Build history of the part. All positions in model axes, mm. Face numbers are marked on the shaded views. Coordinates: 2 decimals unless noted, no trailing zeros.
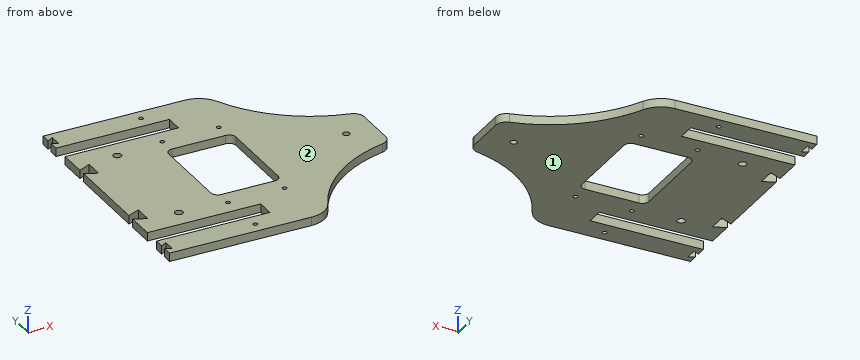
Autodesk Inventor part; units mm, degrees
ref_plane "YZ Plane" through (0, 0, 0) normal (1, 0, 0) x (0, 1, 0)
ref_plane "XZ Plane" through (0, 0, 0) normal (0, 1, 0) x (-1, 0, 0)
ref_plane "XY Plane" through (0, 0, 0) normal (0, 0, 1) x (1, 0, 0)
sketch "Boceto1" plane through (0, 0, 0) normal (0, 0, 1) x (1, 0, 0)
  line L0 (0.0213, 161.5) -> (84.4213, 161.5)
  line L1 (0.0213, 180) -> (0.0213, 172.7)
  line L2 (0.0213, 161.5) -> (0.0213, 168.8)
  line L3 (4.5413, 170.75) -> (4.5413, 175.3)
  line L4 (4.5413, 175.3) -> (0.0213, 172.7)
  line L5 (4.5413, 170.75) -> (4.5413, 166.2)
  line L6 (4.5413, 166.2) -> (0.0213, 168.8)
  line L7 (0.0213, 161.5) -> (84.4213, 161.5)
  line L8 (84.4213, 161.5) -> (84.4213, 148.5)
  line L9 (84.4213, 148.5) -> (0.0213, 148.5)
  line L10 (0.0213, 148.5) -> (0.0213, 127.5)
  line L11 (9.1213, 124.95) -> (9.1213, 131.75)
  line L12 (9.1213, 131.75) -> (0.0213, 127.5)
  line L13 (9.1213, 124.95) -> (9.1213, 118.15)
  line L14 (9.1213, 118.15) -> (0.0213, 122.4)
  line L15 (0.0213, 122.4) -> (0.0213, 90)
  line L16 (0.0213, 180) -> (105.7213, 180)
  line L17 (200.0213, 90) -> (200.0213, 105.2)
  arc A0 (200.0213, 105.2) -> (193.7585, 113.0091) centre (192.0213, 105.2) ccw
  arc A1 (123.7591, 168.6393) -> (105.7213, 180) centre (105.7213, 160) ccw
  arc A2 (123.7591, 168.6393) -> (193.7585, 113.0091) centre (215.9584, 212.7984) ccw
  line L18 (62.2213, 90) -> (62.2213, 120)
  line L19 (112.2213, 120) -> (112.2213, 90)
  circle A3 centre (178.7213, 90) radius 2.5
  circle A4 centre (31.1213, 133.75) radius 3
  line L20 (67.2213, 125) -> (87.2213, 125)
  arc A5 (67.2213, 125) -> (62.2213, 120) centre (67.2213, 120) ccw
  circle A6 centre (66.2213, 136.75) radius 1.65
  circle A7 centre (108.2213, 136.75) radius 1.65
  circle A8 centre (68.5213, 171.35) radius 1.65
  line L21 (87.2213, 125) -> (107.2213, 125)
  arc A9 (112.2213, 120) -> (107.2213, 125) centre (107.2213, 120) ccw
  line L22 (0.0213, 18.5) -> (84.4213, 18.5)
  line L23 (0.0213, 0) -> (0.0213, 7.3)
  line L24 (0.0213, 18.5) -> (0.0213, 11.2)
  line L25 (4.5413, 9.25) -> (4.5413, 4.7)
  line L26 (4.5413, 4.7) -> (0.0213, 7.3)
  line L27 (4.5413, 9.25) -> (4.5413, 13.8)
  line L28 (4.5413, 13.8) -> (0.0213, 11.2)
  line L29 (0.0213, 18.5) -> (84.4213, 18.5)
  line L30 (84.4213, 18.5) -> (84.4213, 31.5)
  line L31 (84.4213, 31.5) -> (0.0213, 31.5)
  line L32 (0.0213, 31.5) -> (0.0213, 52.5)
  line L33 (9.1213, 55.05) -> (9.1213, 48.25)
  line L34 (9.1213, 48.25) -> (0.0213, 52.5)
  line L35 (9.1213, 55.05) -> (9.1213, 61.85)
  line L36 (9.1213, 61.85) -> (0.0213, 57.6)
  line L37 (0.0213, 57.6) -> (0.0213, 90)
  line L38 (0.0213, 0) -> (105.7213, 0)
  line L39 (200.0213, 90) -> (200.0213, 74.8)
  arc A10 (193.7585, 66.9909) -> (200.0213, 74.8) centre (192.0213, 74.8) ccw
  arc A11 (105.7213, 0) -> (123.7591, 11.3607) centre (105.7213, 20) ccw
  arc A12 (193.7585, 66.9909) -> (123.7591, 11.3607) centre (215.9584, -32.7984) ccw
  line L40 (62.2213, 90) -> (62.2213, 60)
  line L41 (112.2213, 60) -> (112.2213, 90)
  circle A13 centre (178.7213, 90) radius 2.5
  circle A14 centre (31.1213, 46.25) radius 3
  line L42 (67.2213, 55) -> (87.2213, 55)
  arc A15 (62.2213, 60) -> (67.2213, 55) centre (67.2213, 60) ccw
  circle A16 centre (66.2213, 43.25) radius 1.65
  circle A17 centre (108.2213, 43.25) radius 1.65
  circle A18 centre (68.5213, 8.65) radius 1.65
  line L43 (87.2213, 55) -> (107.2213, 55)
  arc A19 (107.2213, 55) -> (112.2213, 60) centre (107.2213, 60) ccw
  point P0 (0, 0)
extrude "Extrusión1" add sketch "Boceto1" along normal blind 6.35
fillet "Empalme1" radius 0.01 26 edges at (116.38, 176.9231, 0) (152.3544, 132.7655, 0) (198.2622, 110.2051, 0) (200.0213, 97.6, 0) (198.2622, 69.7949, 0) (152.3544, 47.2345, 0) (116.38, 3.0769, 0) (52.8713, 0, 0) (52.8713, 180, 0) (116.38, 176.9231, 6.35) (152.3544, 132.7655, 6.35) (198.2622, 110.2051, 6.35) (200.0213, 97.6, 6.35) (198.2622, 69.7949, 6.35) (152.3544, 47.2345, 6.35) (116.38, 3.0769, 6.35) (52.8713, 0, 6.35) (52.8713, 180, 6.35) (0.0213, 180, 3.175) (0.0213, 138, 6.35) (0.0213, 138, 0) (0.0213, 106.2, 6.35) (0.0213, 106.2, 0) (0.0213, 42, 6.35) (0.0213, 42, 0) (4.5413, 6.975, 0)
sketch "Boceto2" plane through (0, 0, 6.35) normal (0, 0, 1) x (1, 0, 0)
  point P0 (0, 0)
properties part number "amir"
(1) Probe L1, parallel to Y at x = 48, z = 3; L2, parallel to Y at x = 74, z = 3.5; L3, parallel to X at y = 96.5, z = 4.5. List the from-to ranges inside material, lowest first.
(2) Slice it at C-C, the plane x = 43.5. Give the number of separate pieces and of enclosed holes in the cut face, and give its area (3 significant figures).
(3) Flat gauge pins, fed straight in: P1, Ø2.5, axis at x = 108.22, y = 43.25, coming from the +Z side; P2, Ø1.9, axis at y = 153.5, z = 2.5, coming from the -X side; P3, Ø1.9, axis at y = 55.5, z = 4, coming from the -X side; P4, Ø1, axis at y = 57.5, z = 2.5, coming from the +X side. Where does each tip first touch, or does it go through?
(4) Two-plate mould, pull along Z, no slides. Class the marked faces 1 and 2: pulls with the +Z half, pulls with the -Z half, needs draft (parallel to the pull), parting line crosses it, or undercut.
Results:
1. L1: y = 0 to 18.5, 31.5 to 148.5, 161.5 to 180
1. L2: y = 0 to 18.5, 31.5 to 55, 125 to 148.5, 161.5 to 180
1. L3: x = 0.02 to 62.22, 112.22 to 200.02
2. separate pieces: 3
2. enclosed holes: 0
2. area: 978 mm2
3. P1: passes through
3. P2: stops at x = 84.42
3. P3: stops at x = 9.12
3. P4: stops at x = 168.99
4. face 1: pulls with the -Z half
4. face 2: pulls with the +Z half
